Source: CAD feature listing. Evaluate the final solid. Frame: model axes, mm. Round coordinates to 2 decimals unless told otherwise and drop trailing zeros. Loops run counter-clockwise (first coordinate to the right, second up) from the corner with the lowest first, then second, coordinate; pieces in that order, holes last.
Item 1: First-contact query: P1, Ø2, axis at x = -21.5, z = 2.5, coming from the +Y side; P2, Ø1.5, axis at x = 2.5, z = 2.5, coming from the +Y side; P3, Ø2, axis at y = -41.5, z = 2.5, coming from the -X side. Flat tips, straight axial feed; report the tip coordinate or a pass-through.
Item 2: Section query D-D on x = 53. Return loops of the section in (y, z).
Item 3: Section query C-C on y = 12.5. Return loops of the section in (x, z), then the cut area to 3 significant figures.
Item 4: Section query B-B on x = 0. Return loops of the section in (y, z), then the cut area to 3 significant figures.
Item 5: Section query A-A on y = 0. Return loops of the section in (x, z).
Item 6: Pull-direction query (X, two-part tool) for faces 1 (the cylindrical face through (-59.94, 2.64, 2.46)), 2 (the flat face through (12, 1, 5)), 3 (the cylindrical face through (34.43, -38.74, 2.47)); classes: released by +X, released by -X, zero draft, split by the parting line, or undercut.
Item 7: Ray query, L1, parallel to Y at x = 38.5, z = 4; L2, parallel to Y at x = 53, z = 3.5; L3, parallel to X at y = 52, z = 3.15. Return the intervals inside material, ascending.
```python
from build123d import *

# Parameters (mm, degrees)
SKETCH1_R               = 60
BOSS_EXTRUDE1_DEPTH     = 5
SKETCH7_R               = 10
CUT_EXTRUDE1_DEPTH      = 1
CUT_EXTRUDE1_DEPTH_BACK = 6
M3_CLEARANCE_HOLE1_D    = 3.4
M6_CLEARANCE_HOLE1_D    = 6.6


with BuildPart() as part:
    # Sketch1 → Boss-Extrude1 (new body)
    with BuildSketch(Plane.XY):
        Circle(SKETCH1_R)
    extrude(amount=BOSS_EXTRUDE1_DEPTH)

    # Sketch7 → Cut-Extrude1 (cut, two sides)
    with BuildSketch(Plane.XY.offset(5)) as cut_extrude1_sk:
        Circle(SKETCH7_R)
    extrude(amount=CUT_EXTRUDE1_DEPTH, mode=Mode.SUBTRACT)
    extrude(cut_extrude1_sk.sketch, amount=-CUT_EXTRUDE1_DEPTH_BACK, mode=Mode.SUBTRACT)

    # M3 Clearance Hole1 (through all)
    with Locations(Plane.XY.offset(5)):
        with Locations((0, 12.5), (0, -12.5)):
            Hole(M3_CLEARANCE_HOLE1_D / 2)

    # M6 Clearance Hole1 (through all)
    with Locations(Plane.XY.offset(5)):
        with Locations((-37.476659403, 37.476659403), (0, 53), (37.476659403, 37.476659403), (53, 0), (37.476659403, -37.476659403), (0, -53), (-37.476659403, -37.476659403), (-53, 0)):
            Hole(M6_CLEARANCE_HOLE1_D / 2)


solid = part.part
```
Data:
1. P1: stops at y = 56.39
1. P2: stops at y = 59.97
1. P3: stops at x = -44.27
2. outline: (-28.12, 0) - (-3.3, 0) - (-3.3, 5) - (-28.12, 5) - close; (3.3, 0) - (28.12, 0) - (28.12, 5) - (3.3, 5) - close
3. outline: (-58.68, 0) - (-1.7, 0) - (-1.7, 5) - (-58.68, 5) - close; (1.7, 0) - (58.68, 0) - (58.68, 5) - (1.7, 5) - close
3. area: 570 mm2
4. outline: (-60, 0) - (-56.3, 0) - (-56.3, 5) - (-60, 5) - close; (-49.7, 0) - (-14.2, 0) - (-14.2, 5) - (-49.7, 5) - close; (-10.8, 0) - (-10, 0) - (-10, 5) - (-10.8, 5) - close; (10, 0) - (10.8, 0) - (10.8, 5) - (10, 5) - close; (14.2, 0) - (49.7, 0) - (49.7, 5) - (14.2, 5) - close; (56.3, 0) - (60, 0) - (60, 5) - (56.3, 5) - close
4. area: 400 mm2
5. outline: (-60, 0) - (-56.3, 0) - (-56.3, 5) - (-60, 5) - close; (-49.7, 0) - (-10, 0) - (-10, 5) - (-49.7, 5) - close; (10, 0) - (49.7, 0) - (49.7, 5) - (10, 5) - close; (56.3, 0) - (60, 0) - (60, 5) - (56.3, 5) - close
6. face 1: split by the parting line
6. face 2: zero draft
6. face 3: undercut
7. L1: y = -46.02 to -40.61, -34.34 to 34.34, 40.61 to 46.02
7. L2: y = -28.12 to -3.3, 3.3 to 28.12
7. L3: x = -29.93 to -3.14, 3.14 to 29.93
